Here's how the part is built. I have some questions about the finished solid (model axes, mm). A direction names the side the tool comes from. Round coordinates to 2 decimals unless told otherwise and drop trailing zeros. Write each loop counter-clockwise with the first axis right and the second up, starting at its lowest first coordinate (ties: lowest second). Pieces come first, ordered by that corner, then holes. Notation, with made-up numbers: (38, 22) - (83, 22) arc R18 ccw to (83, 37) - close; hole circle Ø7 at (37.25, 38). An arc over 180 degrees is marked (long way). Use one line per item in the form item = value. Start each with the question number.
1. I want a section at A-A, the plane y = -14.5. List the corners of the cut face in (x, z) for me, plus the area to 3 significant figures.
2. We'd pull the mould along Z, two halves only. Please class faces 1 (the cylindrical face through (-31.35, 45.19, 114.12)), 2 (the cylindrical face through (-36.5, 34.17, -161.23)), 3 (the flat face through (-49, 12, -260.526)), 4 (the flat face through (-1, 0, 239.474)): +Z half, -Z half, draft (parallel to the pull), parting line (faces both ways), or undercut.
3. Which directions (+Z, -Z, +X, -X, +Y, -Y) give clear straight access to the entire face, cutting with the end or side of a thin tool? Please do faces 5 (the flat face through (50, -37, -56)), 6 (the cylindrical face through (-31.35, 45.19, -235.88)), 7 (the flat face through (-41, 29, 139.474)), 8 (the cylindrical face through (-36.5, 34.17, 38.77)), 9 (the flat face through (25, -50, -160)).
4. If I drill on line 1 along Z through (x, y) = (51.5, 9.5); line 2 along Y through (x, z) = (7.5, 63.5); line 3 along X through (y, z) = (1.5, -321), over which ranges is the centre line in solid material (lowest first)?
5. I want a section at B-B, the plane x = -45. List the corners of the cut face in (y, z) for me.
6. Will these pins go through, and if not, where does the flat tip stop? pin 1 (25 mm diameter, centred on x = 29, z = -229, fed in from -Y); pin 2 (8 mm diameter, centred on y = -13.5, z = -133.5, fed in from -X); pin 3 (5 mm diameter, centred on y = -1, z = 126.5, fed in from +X).
7. I want a section at C-C, the plane z = 72.5. List the corners of the cut face in (x, y) for me.
```python
from build123d import *

# Parameters (mm, degrees)
F3_DEPTH = 50
F4_R     = 5
F5_DEPTH = 50


with BuildPart() as f1:
    # F0 (on Right) → F1 (revolve)
    with BuildSketch(Plane.YZ):
        Polygon((-50, -360.526346), (0, -360.526346), (0, 239.473654), (-50, 239.473654), (-50, 139.473654), (-55, 139.473654), (-55, 89.473654), (-50, 89.473654), (-50, -10.526346), (-60, -10.526346), (-60, -110.526346), (-50, -110.526346), (-50, -210.526346), (-55, -210.526346), (-55, -260.526346), (-50, -260.526346), align=None)
    revolve(axis=Axis((0, 0, -60.526346), (0, 0, -1)))

    # F2 (on face) → F3 (cut)
    with BuildSketch(Plane.XY.offset(239.473654)):
        with BuildLine():
            Line((7.5, 41.4343), (7.5, 49.4343))
            ThreePointArc((7.5, 49.4343), (0, 50), (-7.5, 49.4343))
            Line((-7.5, 49.4343), (-7.5, 41.4343))
            Line((-7.5, 41.4343), (7.5, 41.4343))
        make_face()
    extrude(amount=-F3_DEPTH, mode=Mode.SUBTRACT)

    # F4
    f4_edges = [f1.edges().sort_by_distance(p)[0] for p in [
        (-7.5, 45.4343, 189.473654),
        (7.5, 45.4343, 189.473654),
    ]]
    fillet(f4_edges, radius=F4_R)

    # F0 (on Right) → F5 (join)
    with BuildSketch(Plane.YZ):
        Polygon((-50, -360.526346), (0, -360.526346), (0, 239.473654), (-50, 239.473654), (-50, 139.473654), (-55, 139.473654), (-55, 89.473654), (-50, 89.473654), (-50, -10.526346), (-60, -10.526346), (-60, -110.526346), (-50, -110.526346), (-50, -210.526346), (-55, -210.526346), (-55, -260.526346), (-50, -260.526346), align=None)
    extrude(amount=F5_DEPTH)


solid = f1.part
```
Model answer:
q1.outline = (-58.22, -110.53) - (-47.85, -110.53) - (-47.85, -210.53) - (-53.05, -210.53) - (-53.05, -260.53) - (-47.85, -260.53) - (-47.85, -360.53) - (50, -360.53) - (50, -260.53) - (53.05, -260.53) - (53.05, -210.53) - (50, -210.53) - (50, -110.53) - (58.22, -110.53) - (58.22, -10.53) - (50, -10.53) - (50, 89.47) - (53.05, 89.47) - (53.05, 139.47) - (50, 139.47) - (50, 239.47) - (-47.85, 239.47) - (-47.85, 139.47) - (-53.05, 139.47) - (-53.05, 89.47) - (-47.85, 89.47) - (-47.85, -10.53) - (-58.22, -10.53) - close
q1.area = 61,400 mm2
q2.face_1 = draft
q2.face_2 = undercut
q2.face_3 = -Z half
q2.face_4 = +Z half
q3.face_5 = +X, -Y
q3.face_6 = -Z
q3.face_7 = +Z
q3.face_8 = none
q3.face_9 = +X, -X, -Y
q4.line_1 = -260.53 to -210.53, -110.53 to -10.53, 89.47 to 139.47
q4.line_2 = -50 to 49.43
q4.line_3 = -49.98 to 49.98
q5.outline = (-39.69, -110.53) - (-21.79, -110.53) - (-21.79, -210.53) - (-31.62, -210.53) - (-31.62, -260.53) - (-21.79, -260.53) - (-21.79, -360.53) - (21.79, -360.53) - (21.79, -260.53) - (31.62, -260.53) - (31.62, -210.53) - (21.79, -210.53) - (21.79, -110.53) - (39.69, -110.53) - (39.69, -10.53) - (21.79, -10.53) - (21.79, 89.47) - (31.62, 89.47) - (31.62, 139.47) - (21.79, 139.47) - (21.79, 239.47) - (-21.79, 239.47) - (-21.79, 139.47) - (-31.62, 139.47) - (-31.62, 89.47) - (-21.79, 89.47) - (-21.79, -10.53) - (-39.69, -10.53) - close
q6.pin_1 = -55
q6.pin_2 = -49.09
q6.pin_3 = 55
q7.outline = (0, -50) - (50, -50) - (50, 0) arc R50 ccw (long way) to start
